Study the drawing (mm; zero at the part's minimum x, y, z) and answer. A direction names the side the tool comes from. Give positions to 0.01 mm unless a question says otherwise; leave off trailing zeros. Order: outer loops, then holes, each group sorted by start corner. A loop starts at its lowest first (then second) coordinate and runs counter-clockwise, first axis right, second up.
Item 1: Given pin 1 Ø1.5 at (x, y) = (7.5, 2) entering from +Z; pin 2 Ø1 at (y, z) = (9.5, 5.5) entering from -X (1 decimal); pin 3 Ø2 at (y, z) = (10, 2.5) entering from -X, each flat-ended and moving along its own axis, determine where each tip first touches the part or whether it passes through.
Item 2: A cutting plane is placed at D-D (z = 14). Write down the section's boundary in (x, y) (1 decimal).
Item 3: Which of the six approach directions +Z, -Z, +X, -X, +Y, -Y give full straight-line access (tool end or side, diameter ignored) to the marked faces 1 and 2?
Item 4: A cutting plane is placed at A-A (z = 10). Write down the section's boundary in (x, y).
Item 5: A cutting plane is placed at C-C (y = 3.5). Write down the section's boundary in (x, z).
Item 6: The mould has two halves that part along Z. Classify the marked faces 3, 4 and 5: +Z half, -Z half, draft (parallel to the pull), parting line (faces both ways), or undercut.
Item 7: Find the intervals of material crossed by line 1 along Y through (x, z) = (17.1, 10); line 2 along X through (y, z) = (8, 10); line 3 along X through (y, z) = (4.75, 12.75) (1 decimal), in increasing order.
Item 8: A cutting plane is placed at B-B (x = 10). Write down the section's boundary in (y, z).
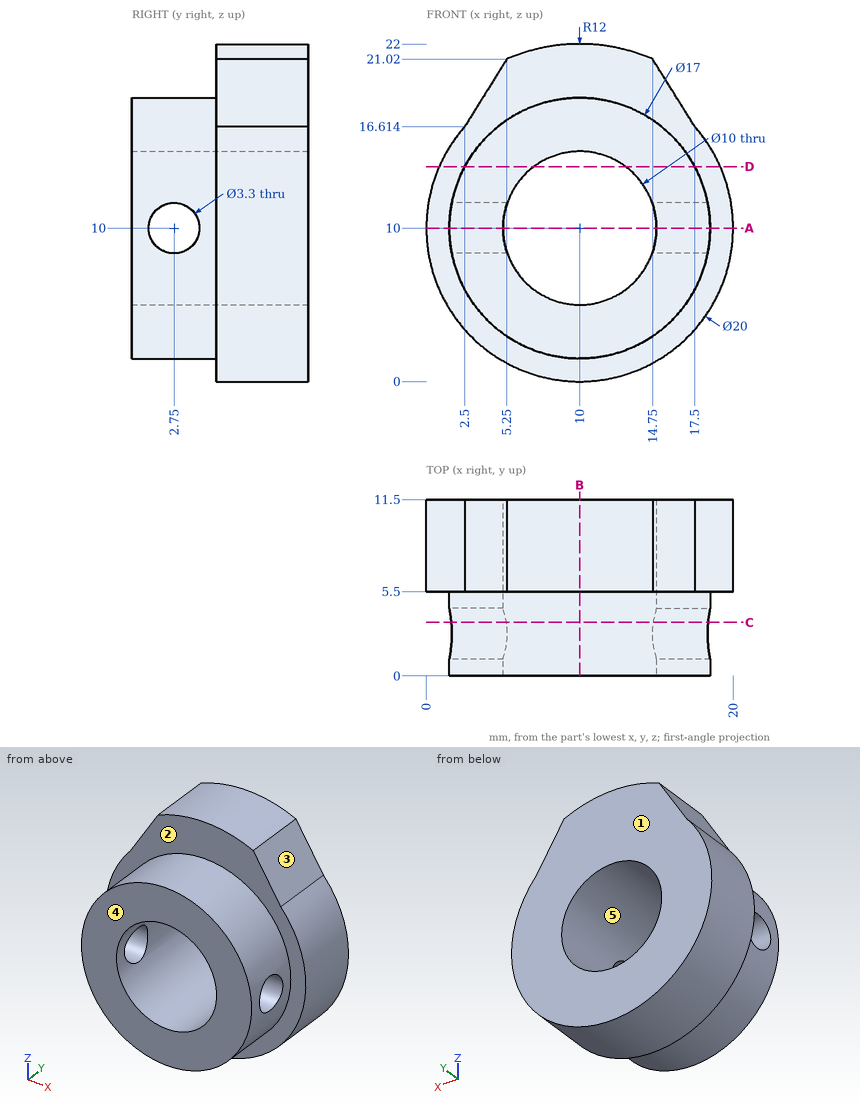
Response values:
1. pin 1: stops at z = 18.32
1. pin 2: stops at x = 0.8
1. pin 3: stops at x = 2.4
2. outline: (0.8, 5.5) - (2.5, 5.5) - (2.5, 0) - (7, 0) - (7, 11.5) - (0.8, 11.5) - close; (13, 0) - (17.5, 0) - (17.5, 5.5) - (19.2, 5.5) - (19.2, 11.5) - (13, 11.5) - close
3. face 1: +Z, -Z, +X, -X, +Y
3. face 2: -Y
4. outline: (0, 5.5) - (1.5, 5.5) - (1.5, 4.4) - (5, 4.4) - (5, 11.5) - (0, 11.5) - close; (1.5, 0) - (5, 0) - (5, 1.1) - (1.5, 1.1) - close; (15, 0) - (18.5, 0) - (18.5, 1.1) - (15, 1.1) - close; (15, 4.4) - (18.5, 4.4) - (18.5, 5.5) - (20, 5.5) - (20, 11.5) - (15, 11.5) - close
5. outline: (1.63, 8.53) arc R8.5 ccw to (18.37, 8.53) - (14.78, 8.53) arc R5 cw to (5.22, 8.53) - close; (1.63, 11.47) - (5.22, 11.47) arc R5 cw to (14.78, 11.47) - (18.37, 11.47) arc R8.5 ccw to start
6. face 3: +Z half
6. face 4: draft
6. face 5: undercut
7. line 1: y = 0 to 1.1, 4.4 to 11.5
7. line 2: x = 0 to 5, 15 to 20
7. line 3: x = 2 to 5.8, 14.2 to 18
8. outline: (0, 1.5) - (5.5, 1.5) - (5.5, 0) - (11.5, 0) - (11.5, 5) - (0, 5) - close; (0, 15) - (11.5, 15) - (11.5, 22) - (5.5, 22) - (5.5, 18.5) - (0, 18.5) - close
